The listing builds one solid part. Answer for the finished solid, in the listing's coordinates (mm). Face numbers are marked on the shaded views. A direction names the side the tool comes from. Coordinates: 2 decimals unless noted, no trailing zeros. Loops run counter-clockwise (first coordinate to the right, second up) from the corner with the lowest first, then second, coordinate; pieces in that order, holes last. Notation, with made-up numbers: (39, 77.5) - (89, 77.5) arc R33 cw to (89, 115.5) - close; hole circle Ø11 at (40, -39.75). An arc over 180 degrees is marked (long way). Return JSON: item names as keys, results as strings. Group by question number.
1. Section D-D (y = 17.5) is taken. Write down the section's boundary in (x, z), and give its area (3 significant figures).
2. Section B-B (z = 11.25) is taken. State how many separate pieces and enclosed holes the cut face has, and give its area (3 significant figures).
3. Which of the six approach directions +Z, -Z, +X, -X, +Y, -Y give full straight-line access (tool end or side, diameter ignored) to the marked faces 4, 5, 6 and 7?
4. Each of these flat-tipped pins is pushed along its axis until it touches: P1, Ø8, axis at x = 30.3, y = 17.5, coming from the -Z side; P2, Ø1.5, axis at y = 4, z = 11, coming from the -X side; P3, Ø6, axis at y = -4, z = 6.5, coming from the -X side. Where does it stop, or does it pass through?
5. Find the intervals of material crossed by line 1 along X through (y, z) = (-3, 1); line 2 along Y through (x, z) = (-13, 11); line 3 along Y through (x, z) = (-7, 6), in increasing order.
6. The mould has two halves that part along Y. Classify the marked faces 1, 2 and 3: pulls with the +Y half, pulls with the -Y half, needs draft (parallel to the pull), parting line crosses it, or undercut.
7. Section C-C (y = -35) is taken. Write down the section's boundary in (x, z), and give its area (3 significant figures).
8. Section A-A (x = 25) is taken. Write down the section's boundary in (y, z), and give its area (3 significant figures).
```python
from build123d import *

# Parameters (mm, degrees)
ESTRUSIONE_ESTRUSIONE1_DEPTH = 15
ESTRUSIONE_ESTRUSIONE5_DEPTH = 0.3
TAGLIO_ESTRUSIONE1_DEPTH     = 16.3
TAGLIO_ESTRUSIONE2_DEPTH     = 16
ESTRUSIONE_ESTRUSIONE2_DEPTH = 5
SCHIZZO7_R                   = 6
TAGLIO_ESTRUSIONE3_DEPTH     = 7


with BuildPart() as part:
    # Schizzo1 → Estrusione-Estrusione1 (new body)
    with BuildSketch(Plane.XY):
        with BuildLine():
            Line((-5.811411188, 38), (-12.489995997, 38))
            ThreePointArc((-12.489995997, 38), (-16.909196271, 36.250228709), (-21.089648938, 33.988626151))
            Line((-21.089648938, 33.988626151), (-17.322367371, 29.336420856))
            ThreePointArc((-17.322367371, 29.336420856), (-16.844140316, 27.721953377), (-17.647583626, 26.242194881))
            Line((-17.647583626, 26.242194881), (-21.99960101, 22.718000691))
            ThreePointArc((-21.99960101, 22.718000691), (-23.61406849, 22.239773636), (-25.093826986, 23.043216946))
            Line((-25.093826986, 23.043216946), (-28.861108553, 27.695422241))
            ThreePointArc((-28.861108553, 27.695422241), (-38.449109313, 11.03023087), (-39.153963342, -8.183346174))
            Line((-39.153963342, -8.183346174), (-35.814606143, -13.967282507))
            ThreePointArc((-35.814606143, -13.967282507), (-29.487341226, -17.025), (-30.002912658, -24.033430901))
            Line((-30.002912658, -24.033430901), (-26.663967345, -29.816653826))
            ThreePointArc((-26.663967345, -29.816653826), (0, -40), (26.663967345, -29.816653826))
            Line((26.663967345, -29.816653826), (30.002912658, -24.033430901))
            ThreePointArc((30.002912658, -24.033430901), (29.487341226, -17.025), (35.814606143, -13.967282507))
            Line((35.814606143, -13.967282507), (39.153963342, -8.183346174))
            ThreePointArc((39.153963342, -8.183346174), (34.641016151, 20), (12.489995997, 38))
            Line((12.489995997, 38), (5.811411188, 38))
            ThreePointArc((5.811411188, 38), (0, 34.05), (-5.811411188, 38))
        make_face()
    extrude(amount=ESTRUSIONE_ESTRUSIONE1_DEPTH)

    # Schizzo5 → Estrusione-Estrusione5 (add)
    with BuildSketch(Plane(origin=(0, 0, 0), x_dir=(-1, 0, 0), z_dir=(0, 0, -1))):
        with BuildLine():
            ThreePointArc((0, -27.5), (27.5, 0), (0, 27.5))
            ThreePointArc((0, 27.5), (-27.5, 0), (0, -27.5))
        make_face()
    extrude(amount=ESTRUSIONE_ESTRUSIONE5_DEPTH)

    # Schizzo2 → Taglio-Estrusione1 (cut, through all)
    with BuildSketch(Plane.XY.offset(15)):
        with BuildLine():
            ThreePointArc((-23.150635095, -9.901923789), (-24.248711306, -14), (-20.150635095, -15.098076211))
            ThreePointArc((-20.150635095, -15.098076211), (-19.052558883, -11), (-23.150635095, -9.901923789))
        make_face()
        with BuildLine():
            ThreePointArc((-11.15, 19.312366504), (-10.16173141, 23.000635095), (-13.85, 23.988903685))
            ThreePointArc((-13.85, 23.988903685), (-14.83826859, 20.300635095), (-11.15, 19.312366504))
        make_face()
        with BuildLine():
            ThreePointArc((11.15, 23.988903685), (10.16173141, 20.300635095), (13.85, 19.312366504))
            ThreePointArc((13.85, 19.312366504), (14.83826859, 23.000635095), (11.15, 23.988903685))
        make_face()
        with BuildLine():
            ThreePointArc((26.35, -2.33826859), (27.33826859, 1.35), (23.65, 2.33826859))
            ThreePointArc((23.65, 2.33826859), (22.66173141, -1.35), (26.35, -2.33826859))
        make_face()
        with BuildLine():
            ThreePointArc((13.85, -23.988903685), (14.83826859, -20.300635095), (11.15, -19.312366504))
            ThreePointArc((11.15, -19.312366504), (10.16173141, -23.000635095), (13.85, -23.988903685))
        make_face()
        with BuildLine():
            ThreePointArc((-11.15, -23.988903685), (-10.16173141, -20.300635095), (-13.85, -19.312366504))
            ThreePointArc((-13.85, -19.312366504), (-14.83826859, -23.000635095), (-11.15, -23.988903685))
        make_face()
        with BuildLine():
            ThreePointArc((-23.65, -2.33826859), (-22.66173141, 1.35), (-26.35, 2.33826859))
            ThreePointArc((-26.35, 2.33826859), (-27.33826859, -1.35), (-23.65, -2.33826859))
        make_face()
    extrude(amount=-TAGLIO_ESTRUSIONE1_DEPTH, mode=Mode.SUBTRACT)

    # Schizzo3 → Taglio-Estrusione2 (cut, through all)
    with BuildSketch(Plane(origin=(0, 0, 0), x_dir=(-1, 0, 0), z_dir=(0, 0, -1))):
        with BuildLine():
            ThreePointArc((30.3, 20.9), (26.9, 17.5), (30.3, 14.1))
            ThreePointArc((30.3, 14.1), (33.7, 17.5), (30.3, 20.9))
        make_face()
        with BuildLine():
            ThreePointArc((0, -38.4), (3.4, -35), (0, -31.6))
            ThreePointArc((0, -31.6), (-3.4, -35), (0, -38.4))
        make_face()
        with BuildLine():
            ThreePointArc((-30.3, 20.9), (-33.7, 17.5), (-30.3, 14.1))
            ThreePointArc((-30.3, 14.1), (-26.9, 17.5), (-30.3, 20.9))
        make_face()
    extrude(amount=-TAGLIO_ESTRUSIONE2_DEPTH, mode=Mode.SUBTRACT)

    # Schizzo4 → Estrusione-Estrusione2 (add)
    with BuildSketch(Plane.XY.offset(15)):
        with BuildLine():
            ThreePointArc((-7.875, 13.63990011), (-13.63990011, -7.875), (7.875, -13.63990011))
            ThreePointArc((7.875, -13.63990011), (13.63990011, 7.875), (-7.875, 13.63990011))
        make_face()
    extrude(amount=ESTRUSIONE_ESTRUSIONE2_DEPTH)

    # Schizzo7 → Taglio-Estrusione3 (cut)
    with BuildSketch(Plane(origin=(0, 0, -0.3), x_dir=(-1, 0, 0), z_dir=(0, 0, -1))):
        with Locations((-12.5, 21.650635095)):
            Circle(SCHIZZO7_R)
        with Locations((12.5, 21.650635095)):
            Circle(SCHIZZO7_R)
        with Locations((25, 0)):
            Circle(SCHIZZO7_R)
        with Locations((12.5, -21.650635095)):
            Circle(SCHIZZO7_R)
        with Locations((-12.5, -21.650635095)):
            Circle(SCHIZZO7_R)
        with Locations((-25, 0)):
            Circle(SCHIZZO7_R)
    extrude(amount=-TAGLIO_ESTRUSIONE3_DEPTH, mode=Mode.SUBTRACT)


solid = part.part
```
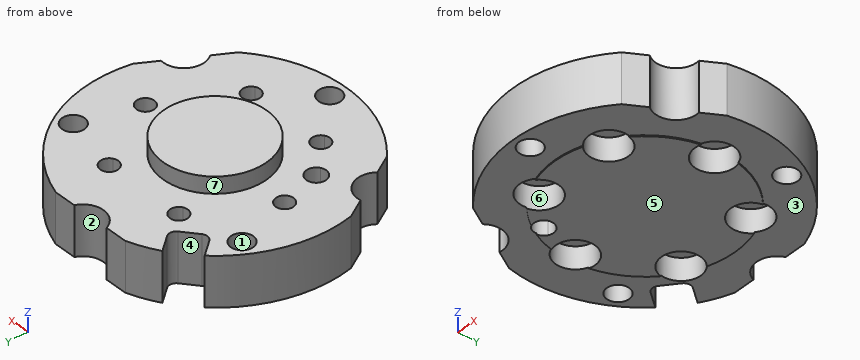
The answers:
{
 "1": {"outline": "(-35.97, 0) - (-33.7, 0) - (-33.7, 15) - (-35.97, 15) - close; (-26.9, 0) - (-21.21, 0) - (-21.21, -0.3) - (-16.83, -0.3) - (-16.83, 6.7) - (-8.17, 6.7) - (-8.17, -0.3) - (8.17, -0.3) - (8.17, 6.7) - (16.83, 6.7) - (16.83, -0.3) - (21.21, -0.3) - (21.21, 0) - (26.9, 0) - (26.9, 15) - (-26.9, 15) - close; (33.7, 0) - (35.97, 0) - (35.97, 15) - (33.7, 15) - close", "area": "766 mm2"},
 "2": {"separate pieces": "1", "enclosed holes": "10", "area": "4,470 mm2"},
 "3": {"face 4": "+Z, -Z", "face 5": "-Z, +X, -X, +Y, -Y", "face 6": "-Z", "face 7": "+Z"},
 "4": {"P1": "stops at z = 0", "P2": "stops at x = -39.87", "P3": "stops at x = -39.99"},
 "5": {"line 1": "x = -39.89 to -30.2, -19.8 to 19.8, 30.2 to 39.89", "line 2": "y = -37.83 to -24.3, -19 to 19, 24.3 to 37.83", "line 3": "y = -39.38 to -24.05, -19.25 to 19.25, 24.05 to 38"},
 "6": {"face 1": "undercut", "face 2": "pulls with the +Y half", "face 3": "needs draft"},
 "7": {"outline": "(-19.36, 0) - (-3.4, 0) - (-3.4, 15) - (-19.36, 15) - close; (3.4, 0) - (19.36, 0) - (19.36, 15) - (3.4, 15) - close", "area": "479 mm2"},
 "8": {"outline": "(-31.22, 0) - (-11.46, 0) - (-11.46, -0.3) - (-6, -0.3) - (-6, 6.7) - (-2.7, 6.7) - (-2.7, 15) - (-31.22, 15) - close; (2.7, 6.7) - (6, 6.7) - (6, -0.3) - (11.46, -0.3) - (11.46, 0) - (31.22, 0) - (31.22, 15) - (2.7, 15) - close", "area": "815 mm2"}
}
